Study the drawing (mm; zero at the part's minimum x, y, z) and answer. A direction names the side the tool comes from. Give positions to 0.01 mm unless a question says otherwise; leave off trailing zeros. Write each loop counter-clockwise with the first axis right and the second up, starting at its lowest first coordinate (ties: lowest second). Pieces come first, ordered by that corner, then holes. Notation, with made-up numbers: (40, -28.75) -> (54, -28.75) arc R28 ccw to (54, 9.25) -> close; hole circle Ø10 at (26.5, 80.5). An arc over 180 degrees is marked (long way). Put each result on its own line as item: value. Start each with the question number.
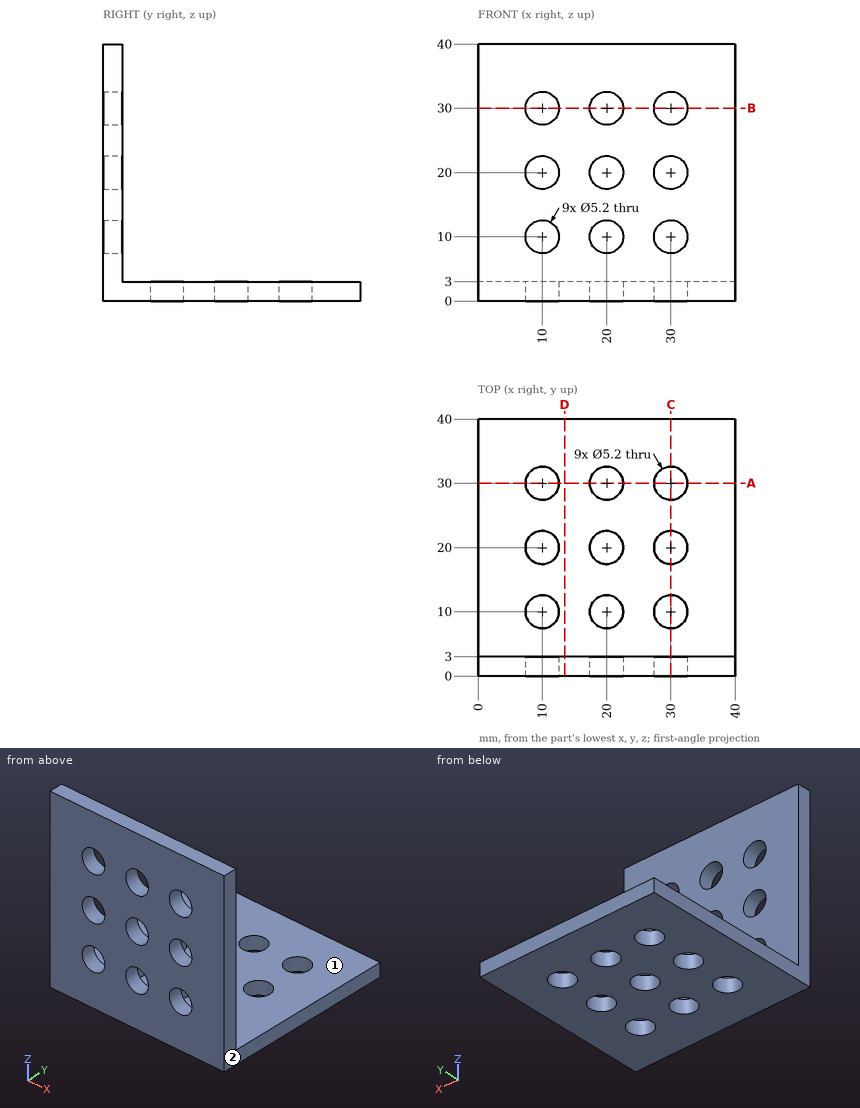
1) Each of these flat-tipped pins is pushed along its axis until it touches: pin 1 Ø7 at (x, z) = (20, 30) entering from +Y; pin 2 Ø10 at (x, y) = (15.5, 11) entering from +Z. Where does it stop, or does it pass through?
2) A cutting plane is placed at C-C on x = 30. State how many separate pieces and enclosed holes the cut face has, and give its area (3 significant figures).
3) A cutting plane is placed at D-D on x = 13.5. Give the vertices of the cut face in (y, z), and give its area (3 significant figures).
4) A cutting plane is placed at A-A on y = 30. Give the vertices of the cut face in (x, z).
5) For the marked faces 1 and 2, determine the directions among +Z, -Z, +X, -X, +Y, -Y from which every point of the face is accessible in a straight line to the end or side of a thin tool.
6) A straight line is drawn through the part: line 1 (X direction, y = 1.65, z = 10). Find the intervals that lie inside material, in ascending order. Write a range as [from, to].
Results found:
1. pin 1: stops at y = 3
1. pin 2: stops at z = 3
2. separate pieces: 7
2. enclosed holes: 0
2. area: 137 mm²
3. outline: (0, 0) -> (40, 0) -> (40, 3) -> (3, 3) -> (3, 40) -> (0, 40) -> close
3. area: 231 mm²
4. outline: (0, 0) -> (7.4, 0) -> (7.4, 3) -> (0, 3) -> close; (12.6, 0) -> (17.4, 0) -> (17.4, 3) -> (12.6, 3) -> close; (22.6, 0) -> (27.4, 0) -> (27.4, 3) -> (22.6, 3) -> close; (32.6, 0) -> (40, 0) -> (40, 3) -> (32.6, 3) -> close
5. face 1: +Z, +X, -X, +Y
5. face 2: +Z, -Z, +X, +Y, -Y
6. line 1: x = [0, 7.4], [12.6, 17.4], [22.6, 27.4], [32.6, 40]
